Verification items for the finished model (mm, model axes). Face numbers are marked on the shaded views. Round coordinates to 2 decimals unless told otherwise and drop trailing zeros. Order: outer loops, then holes, each group sorted by start corner. A loop starts at its lowest first (then second) coordinate and runs counter-clockwise, first axis right, second up. Notation, with made-up numbers: (61, -10.75) -> (99, -10.75) arc R26 ccw to (99, 4.25) -> close; hole circle Ø9 at (41.25, -33). An arc over 180 degrees is marked (long way). Answer in a Markdown table with one row per item. Add a question column.
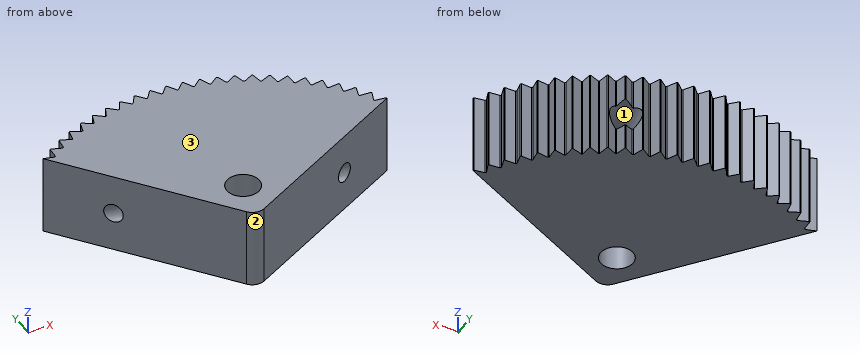
```python
from build123d import *

# Parameters (mm, degrees)
SKETCH1_R                = 1.3
BOSS_EXTRUDE1_DEPTH      = 3.175
BOSS_EXTRUDE1_DEPTH_BACK = 3.175
SKETCH4_R                = 0.75
SKETCH3_R                = 1.1303
CUT_EXTRUDE2_DEPTH       = 7.5
CUT_EXTRUDE2_DEPTH_BACK  = 10
CUT_EXTRUDE3_DEPTH       = 10
CUT_EXTRUDE3_DEPTH_BACK  = 10


with BuildPart() as part:
    # Sketch1 → Boss-Extrude1 (new body, two sides)
    with BuildSketch(Plane.XY) as boss_extrude1_sk:
        with BuildLine():
            Line((-19.351944596, 11.121666082), (-9.732209918, -1.193299023))
            ThreePointArc((-9.732209918, -1.193299023), (-9.152143222, -1.55583694), (-8.474751471, -1.460697412))
            Line((-8.474751471, -1.460697412), (5.323571039, 5.874420633))
            ThreePointArc((5.323571039, 5.874420633), (-5.801036197, 14.202963476), (-19.351944596, 11.121666082))
        make_face()
        with Locations((-8.471265065, 1.646037216)):
            Circle(SKETCH1_R, mode=Mode.SUBTRACT)
    extrude(amount=BOSS_EXTRUDE1_DEPTH)
    extrude(boss_extrude1_sk.sketch, amount=-BOSS_EXTRUDE1_DEPTH_BACK)

    # Cut-Sweep1: sweep along a path in Sketch2
    with BuildLine(Plane.XY) as cut_sweep1_path:
        Line((-16.021378593, 6.857951387), (3.426511905, 2.722359798))
    # Sketch4 → Cut-Sweep1 (sweep, cut)
    with BuildSketch(Plane(origin=(-6.623066075, -5.173554115, 0), x_dir=(0, 0, 1), z_dir=(-0.788065719, -0.615591117, 0))):
        with Locations((0, 15.267134729)):
            Circle(SKETCH4_R)
    sweep(path=cut_sweep1_path.line, mode=Mode.SUBTRACT)

    # Sketch3 → Cut-Extrude2 (cut, two sides)
    with BuildSketch(Plane(origin=(2.63861758, 12.40827211, 0), x_dir=(0.978129034, -0.207999022, 0), z_dir=(-0.207999022, -0.978129034, 0))) as cut_extrude2_sk:
        with Locations((-5.633213298, 0)):
            Circle(SKETCH3_R)
    extrude(amount=CUT_EXTRUDE2_DEPTH, mode=Mode.SUBTRACT)
    extrude(cut_extrude2_sk.sketch, amount=-CUT_EXTRUDE2_DEPTH_BACK, mode=Mode.SUBTRACT)

    # Sketch5 → Cut-Extrude3 (cut, two sides)
    with BuildSketch(Plane.XY) as cut_extrude3_sk:
        with BuildLine():
            Line((-18.335959881, 11.845477975), (-17.532299102, 11.545639171))
            Line((-17.532299102, 11.545639171), (-17.446850408, 11.59758646))
            Line((-17.446850408, 11.59758646), (-17.343115269, 12.449063399))
            ThreePointArc((-17.343115269, 12.449063399), (-17.844834345, 12.155983405), (-18.335959881, 11.845477975))
        make_face()
        with BuildLine():
            Line((-19.351944596, 11.121666082), (-18.527988766, 10.883190202))
            Line((-18.527988766, 10.883190202), (-18.446694016, 10.941423901))
            Line((-18.446694016, 10.941423901), (-18.407365445, 11.798294498))
            ThreePointArc((-18.407365445, 11.798294498), (-18.88559278, 11.468269454), (-19.351944596, 11.121666082))
        make_face()
        with BuildLine():
            Line((-17.268359717, 12.490736443), (-16.489556709, 12.131237025))
            Line((-16.489556709, 12.131237025), (-16.400439201, 12.176602977))
            Line((-16.400439201, 12.176602977), (-16.23288644, 13.017852066))
            ThreePointArc((-16.23288644, 13.017852066), (-16.755248788, 12.763381061), (-17.268359717, 12.490736443))
        make_face()
        with BuildLine():
            Line((-16.15520532, 13.053778081), (-15.405681675, 12.636659079))
            Line((-15.405681675, 12.636659079), (-15.313401308, 12.675186133))
            Line((-15.313401308, 12.675186133), (-15.082982195, 13.501431247))
            ThreePointArc((-15.082982195, 13.501431247), (-15.623022142, 13.287013969), (-16.15520532, 13.053778081))
        make_face()
        with BuildLine():
            Line((-15.002816533, 13.531406266), (-14.286827611, 13.059035839))
            Line((-14.286827611, 13.059035839), (-14.191908301, 13.090505261))
            Line((-14.191908301, 13.090505261), (-13.89993102, 13.89705546))
            ThreePointArc((-13.89993102, 13.89705546), (-14.454582535, 13.723909246), (-15.002816533, 13.531406266))
        make_face()
        with BuildLine():
            Line((-13.817735952, 13.920909302), (-13.139346723, 13.395969296))
            Line((-13.139346723, 13.395969296), (-13.042327365, 13.42020242))
            Line((-13.042327365, 13.42020242), (-12.690449596, 14.202478581))
            ThreePointArc((-12.690449596, 14.202478581), (-13.256563688, 14.071586455), (-13.817735952, 13.920909302))
        make_face()
        with BuildLine():
            Line((-12.606691776, 14.220075817), (-11.96975374, 13.645546536))
            Line((-11.96975374, 13.645546536), (-11.871185156, 13.662405782))
            Line((-11.871185156, 13.662405782), (-11.461404655, 14.415966594))
            ThreePointArc((-11.461404655, 14.415966594), (-12.035767257, 14.328071685), (-12.606691776, 14.220075817))
        make_face()
        with BuildLine():
            Line((-11.376559612, 14.427207318), (-10.784688934, 13.806350606))
            Line((-10.784688934, 13.806350606), (-10.685130738, 13.815740255))
            Line((-10.685130738, 13.815740255), (-10.219774001, 14.536307437))
            ThreePointArc((-10.219774001, 14.536307437), (-10.799124216, 14.491908762), (-11.376559612, 14.427207318))
        make_face()
        with BuildLine():
            Line((-10.134323437, 14.541127831), (-9.590880415, 13.877468553))
            Line((-9.590880415, 13.877468553), (-9.49089784, 13.879335297))
            Line((-9.49089784, 13.879335297), (-8.972606893, 14.562817887))
            ThreePointArc((-8.972606893, 14.562817887), (-9.553655506, 14.562167515), (-10.134323437, 14.541127831))
        make_face()
        with BuildLine():
            Line((-8.887035946, 14.561190583), (-8.395105934, 13.85849661))
            Line((-8.395105934, 13.85849661), (-8.295266624, 13.852829851))
            Line((-8.295266624, 13.852829851), (-7.726984022, 14.49534743))
            ThreePointArc((-7.726984022, 14.49534743), (-8.306432177, 14.538449054), (-8.887035946, 14.561190583))
        make_face()
        with BuildLine():
            Line((-7.641778514, 14.487281668), (-7.204154406, 13.749542489))
            Line((-7.204154406, 13.749542489), (-7.10502519, 13.736374399))
            Line((-7.10502519, 13.736374399), (-6.489977312, 14.334279127))
            ThreePointArc((-6.489977312, 14.334279127), (-7.064535238, 14.420888041), (-7.641778514, 14.487281668))
        make_face()
        with BuildLine():
            Line((-6.405620991, 14.319820698), (-6.024787362, 13.551224769))
            Line((-6.024787362, 13.551224769), (-5.926931038, 13.530630109))
            Line((-5.926931038, 13.530630109), (-5.268609769, 14.080527429))
            ThreePointArc((-5.268609769, 14.080527429), (-5.835015459, 14.210151917), (-6.405620991, 14.319820698))
        make_face()
        with BuildLine():
            Line((-5.185581561, 14.05975842), (-4.863700563, 13.264669382))
            Line((-4.863700563, 13.264669382), (-4.767672704, 13.236765076))
            Line((-4.767672704, 13.236765076), (-4.06981561, 13.73553299))
            ThreePointArc((-4.06981561, 13.73553299), (-4.624853342, 13.907437121), (-5.185581561, 14.05975842))
        make_face()
        with BuildLine():
            Line((-3.9885869, 13.708571317), (-3.727485988, 12.891503223))
            Line((-3.727485988, 12.891503223), (-3.633831783, 12.856447697))
            Line((-3.633831783, 12.856447697), (-2.900400891, 13.30125449))
            ThreePointArc((-2.900400891, 13.30125449), (-3.440919483, 13.514462291), (-3.9885869, 13.708571317))
        make_face()
        with BuildLine():
            Line((-2.82143285, 13.268253224), (-2.622594402, 12.433844914))
            Line((-2.622594402, 12.433844914), (-2.531845566, 12.391837192))
            Line((-2.531845566, 12.391837192), (-1.767004872, 12.78015751))
            ThreePointArc((-1.767004872, 12.78015751), (-2.289935572, 13.033458511), (-2.82143285, 13.268253224))
        make_face()
        with BuildLine():
            Line((-1.690745835, 12.741304013), (-1.55529874, 11.894292773))
            Line((-1.55529874, 11.894292773), (-1.467970492, 11.84557135))
            Line((-1.467970492, 11.84557135), (-0.676062318, 12.175200535))
            ThreePointArc((-0.676062318, 12.175200535), (-1.178436229, 12.46715664), (-1.690745835, 12.741304013))
        make_face()
        with BuildLine():
            Line((-0.602945237, 12.130715396), (-0.531658487, 11.275910064))
            Line((-0.531658487, 11.275910064), (-0.448246626, 11.220751552))
            Line((-0.448246626, 11.220751552), (0.366233034, 11.489818161))
            ThreePointArc((0.366233034, 11.489818161), (-0.112731901, 11.818771812), (-0.602945237, 12.130715396))
        make_face()
        with BuildLine():
            Line((0.43579304, 11.439953939), (0.442514722, 10.582207604))
            Line((0.442514722, 10.582207604), (0.521536632, 10.520925162))
            Line((0.521536632, 10.520925162), (1.353963634, 10.72790159))
            ThreePointArc((1.353963634, 10.72790159), (0.90112696, 11.091985181), (0.43579304, 11.439953939))
        make_face()
        with BuildLine():
            Line((1.419571645, 10.672941387), (1.361690097, 9.817123835))
            Line((1.361690097, 9.817123835), (1.435873415, 9.750065388))
            Line((1.435873415, 9.750065388), (2.281521722, 9.893776544))
            ThreePointArc((2.281521722, 9.893776544), (1.857384253, 10.290923018), (1.419571645, 10.672941387))
        make_face()
        with BuildLine():
            Line((2.342805254, 9.834032391), (2.220649092, 8.985002457))
            Line((2.220649092, 8.985002457), (2.289572649, 8.912548725))
            Line((2.289572649, 8.912548725), (3.143641161, 8.9921787))
            ThreePointArc((3.143641161, 8.9921787), (2.750610903, 9.42013329), (2.342805254, 9.834032391))
        make_face()
        with BuildLine():
            Line((3.200252281, 8.92798979), (3.014515038, 8.090567774))
            Line((3.014515038, 8.090567774), (3.077787526, 8.013130106))
            Line((3.077787526, 8.013130106), (3.935427337, 8.028226808))
            ThreePointArc((3.935427337, 8.028226808), (3.575735688, 8.484559836), (3.200252281, 8.92798979))
        make_face()
        with BuildLine():
            Line((3.98704464, 7.959957568), (3.738780825, 7.138897866))
            Line((3.738780825, 7.138897866), (3.796043018, 7.056915909))
            Line((3.796043018, 7.056915909), (4.652384947, 7.007393627))
            ThreePointArc((4.652384947, 7.007393627), (4.328074028, 7.489514298), (3.98704464, 7.959957568))
        make_face()
        with BuildLine():
            Line((4.69871538, 6.93543165), (4.38933449, 6.135395762))
            Line((4.38933449, 6.135395762), (4.440261288, 6.049334963))
            Line((4.440261288, 6.049334963), (5.290443523, 5.935474855))
            ThreePointArc((5.290443523, 5.935474855), (5.003354583, 6.440645969), (4.69871538, 6.93543165))
        make_face()
    extrude(amount=CUT_EXTRUDE3_DEPTH, mode=Mode.SUBTRACT)
    extrude(cut_extrude3_sk.sketch, amount=-CUT_EXTRUDE3_DEPTH_BACK, mode=Mode.SUBTRACT)


solid = part.part
```
1) Thickness scan on L1, parallel to Y at x = -7.75, z = -0.25; L2, parallel to Y at x = -0.75, z = -0.5; L3, parallel to Y at x = -13.75, z = 0.5. Record the ranges inside material, lowest first. Write a range as [from, to].
2) Draft check along Z on the marked faces 1, 2 and 3. Enter one of: +Z half, -Z half, draft (parallel to the pull), parting line (faces both ways), or undercut.
3) Depth check by flat-ended pin: P1, Ø1.6, axis at x = -8.47, y = 1.65, coming from the -Z side; P2, Ø1.5, axis at x = 2, z = -2, coming from the -Y side; P3, Ø1.5, axis at x = -16.5, z = -0.5, coming from the -Y side. Enter the tip coordinate at first touch or a pass-through.
4) Cross-section at A-A, the plane y = 1.25. Record the boundary of the cut face in (x, z) (3 decimals).
Results below:
| question | item | result |
|---|---|---|
| 1 | L1 | [-1.08, 0.56], [2.73, 4.63], [5.56, 14.47] |
| 1 | L2 | [2.65, 3.24], [3.98, 12.14] |
| 1 | L3 | [3.95, 6.01], [6.74, 13.87] |
| 2 | face 1 | undercut |
| 2 | face 2 | draft |
| 2 | face 3 | +Z half |
| 3 | P1 | through |
| 3 | P2 | y = 3.71 |
| 3 | P3 | y = 6.52 |
| 4 | outline | (-11.641, -3.175) -> (-9.709, -3.175) -> (-9.709, 3.175) -> (-11.641, 3.175) -> close; (-7.233, -3.175) -> (-3.376, -3.175) -> (-3.376, 3.175) -> (-7.233, 3.175) -> close |
